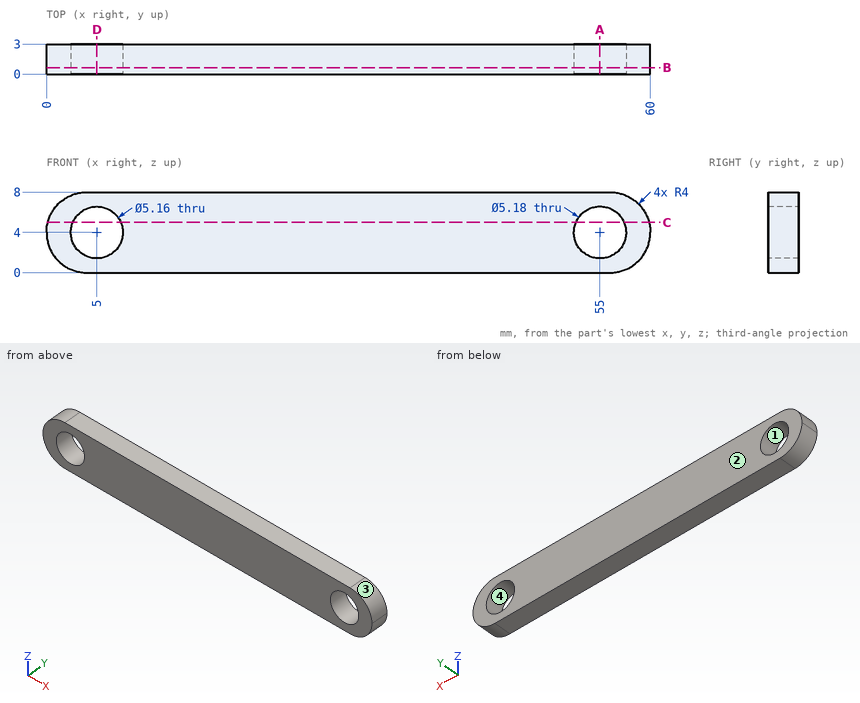
Geometry: see drawing. Coordinates: mm, zero at the bounding-box minimum. Coordinates: 2 decimals unless noted, no trailing zeros. Loops run counter-clockwise (first coordinate to the right, second up) from the corner with the lowest first, then second, coordinate; pieces in that order, holes last. Notation, with made-up numbers: (12.25, -22.75) - (27.25, -22.75) arc R24 cw to (27.25, 10.25) - close; hole circle Ø10 at (56.25, -9.75). An arc over 180 degrees is marked (long way). Return JSON: item names as keys, results as strings.
Q1. Section B-B, the plane y = 0.65. Give the number of separate pieces and of enclosed holes in the cut face, plus the area to 3 significant figures.
Results:
{"separate pieces": "1", "enclosed holes": "2", "area": "424 mm2"}
Q2. Material intervals for line 1 along X through (y, z) = (2.3, 4); line 2 along X through (y, z) = (0.8, 5.75); line 3 along Z through (x, y) = (56, 1.15), sorted ascending.
Results:
{"line 1": "0 to 2.42, 7.58 to 52.41, 57.59 to 60", "line 2": "0.4 to 3.1, 6.9 to 53.09, 56.91 to 59.6", "line 3": "0 to 1.61, 6.39 to 8"}
Q3. Section A-A, the plane x = 55. Return loops of the section in (y, z).
Results:
{"outline": "(0, 0) - (3, 0) - (3, 1.41) - (0, 1.41) - close; (0, 6.59) - (3, 6.59) - (3, 8) - (0, 8) - close"}
Q4. Section D-D, the plane x = 5. Return loops of the section in (y, z).
Results:
{"outline": "(0, 0) - (3, 0) - (3, 1.42) - (0, 1.42) - close; (0, 6.58) - (3, 6.58) - (3, 8) - (0, 8) - close"}
Q5. Section C-C, the plane z = 5. Return loops of the section in (x, y).
Results:
{"outline": "(0.13, 0) - (2.62, 0) - (2.62, 3) - (0.13, 3) - close; (7.38, 0) - (52.61, 0) - (52.61, 3) - (7.38, 3) - close; (57.39, 0) - (59.87, 0) - (59.87, 3) - (57.39, 3) - close"}
Q6. Mould query, pull axis Z, two halves, no side actions, for the marked faces 1, 2, 3 and 4. Classes: released by +Z, released by -Z, zero draft, split by the parting line, or undercut.
Results:
{"face 1": "undercut", "face 2": "zero draft", "face 3": "released by +Z", "face 4": "undercut"}
